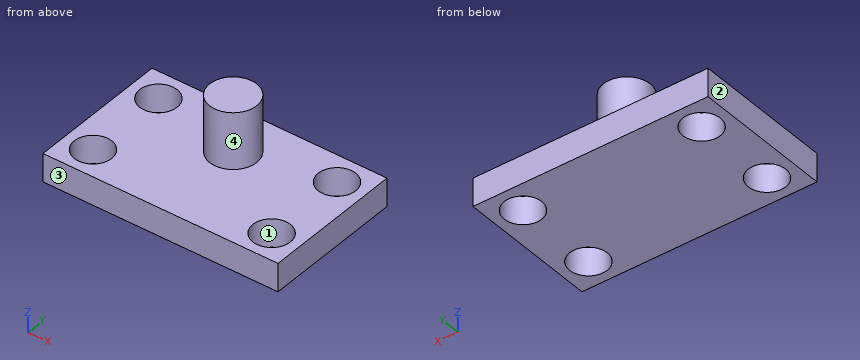
from build123d import *

# Parameters (mm, degrees)
SKETCH1_W           = 250
SKETCH1_H           = 150
SKETCH1_R           = 20
BOSS_EXTRUDE1_DEPTH = 30
SKETCH2_R           = 25
BOSS_EXTRUDE3_DEPTH = 90


with BuildPart() as part:
    # Sketch1 → Boss-Extrude1 (new body)
    with BuildSketch(Plane.XY):
        with Locations((125, 75)):
            Rectangle(SKETCH1_W, SKETCH1_H)
        with Locations((30, 30)):
            Circle(SKETCH1_R, mode=Mode.SUBTRACT)
        with Locations((220, 30)):
            Circle(SKETCH1_R, mode=Mode.SUBTRACT)
        with Locations((220, 120)):
            Circle(SKETCH1_R, mode=Mode.SUBTRACT)
        with Locations((30, 120)):
            Circle(SKETCH1_R, mode=Mode.SUBTRACT)
    extrude(amount=BOSS_EXTRUDE1_DEPTH)

    # Sketch2 → Boss-Extrude3 (add)
    with BuildSketch(Plane.XY):
        with Locations(Location((125, 100, 0), (0, 0, 180))):
            Circle(SKETCH2_R)
    extrude(amount=BOSS_EXTRUDE3_DEPTH)


solid = part.part
Verification items for the finished model (mm, model axes). Face numbers are marked on the shaded views. Give positions to 0.01 mm unless a question says otherwise; leave off trailing zeros. Loops run counter-clockwise (first coordinate to the right, second up) from the corner with the lowest first, then second, coordinate; pieces in that order, holes last.
1) Sectioned sample at B-B, the plane x = 220. Enter the section's corners in (y, z).
2) Sectioned sample at A-A, the plane y = 120. Enter the section's corners in (x, z).
3) Depth check by flat-ended pin: pin 1 Ø12 at (y, z) = (79, 76.5) entering from -X; pin 2 Ø1 at (x, y) = (145.5, 33) entering from +Z; pin 3 Ø12 at (y, z) = (126.5, 37) entering from -X. Enter the tip coordinate at first touch or a pass-through.
4) Thickness scan on line 1 along Y through (x, z) = (220, 18.75); line 2 along Y through (x, z) = (216.5, 8); line 3 along Z through (x, y) = (229, 142.5). Record the ranges inside material, lowest first.
5) Sectioned sample at C-C, the plane x = 125. Enter the section's corners in (y, z), then the cut area to 3 significant figures.
6) Sectioned sample at D-D, the plane z = 12. Enter the section's corners in (x, y), then the cut area to 3 significant figures.
7) Draft check along X on the marked faces 1, 2, 3 and 4. Enter one of: pulls with the +X half, pulls with the -X half, needs draft (parallel to the pull), parting line crosses it, or undercut.
Answers:
1. outline: (0, 0) - (10, 0) - (10, 30) - (0, 30) - close; (50, 0) - (100, 0) - (100, 30) - (50, 30) - close; (140, 0) - (150, 0) - (150, 30) - (140, 30) - close
2. outline: (0, 0) - (10, 0) - (10, 30) - (0, 30) - close; (50, 0) - (200, 0) - (200, 30) - (140, 30) - (140, 90) - (110, 90) - (110, 30) - (50, 30) - close; (240, 0) - (250, 0) - (250, 30) - (240, 30) - close
3. pin 1: stops at x = 105
3. pin 2: stops at z = 30
3. pin 3: stops at x = 110.69
4. line 1: y = 0 to 10, 50 to 100, 140 to 150
4. line 2: y = 0 to 10.31, 49.69 to 100.31, 139.69 to 150
4. line 3: z = 0 to 30
5. outline: (0, 0) - (150, 0) - (150, 30) - (125, 30) - (125, 90) - (75, 90) - (75, 30) - (0, 30) - close
5. area: 7,500 mm2
6. outline: (0, 0) - (250, 0) - (250, 150) - (0, 150) - close; hole circle Ø40 at (30, 30); hole circle Ø40 at (30, 120); hole circle Ø40 at (220, 30); hole circle Ø40 at (220, 120)
6. area: 32,500 mm2
7. face 1: undercut
7. face 2: pulls with the -X half
7. face 3: needs draft
7. face 4: parting line crosses it
